The listing builds one solid part. Answer for the finished solid, in the listing's coordinates (mm). Face numbers are marked on the shaded views. A direction names the side the tool comes from. Give positions to 0.01 mm unless a question says otherwise; leave off trailing zeros. Order: outer loops, then holes, each group sorted by start corner. A loop starts at its lowest first (then second) coordinate and runs counter-clockwise, first axis right, second up. Notation, with made-up numbers: (45, -28.75) - (92, -28.75) arc R13 ccw to (92, -23.75) - close; hole circle Ø8 at (63, 46). An arc over 180 degrees is marked (long way). Use a Markdown table: item, result. Add a question column.
1) Flat-ended cylindrical pins translate along their axes: pin 1 (1 mm diameter, centred on y = 13, z = 19.5, fed in from +X); pin 2 (2.5 mm diameter, centred on x = 11.67, y = 11.67, fed in from -Z); pin 3 (4 mm diameter, centred on x = -11.5, z = 7, fed in from +Y). Find the tip coordinate at first contact, or state that the pin passes through.
2) Find section A-A, the plane z = 42. Determine the outline of the cut face in (x, y), plus the area to 3 significant figures.
3) The mould has two halves that part along Z. Classify the marked faces 4, 5 and 6: released by +Z, released by -Z, zero draft, split by the parting line, or undercut.
4) For the marked faces 1, 2 and 3, determine the directions among +Z, -Z, +X, -X, +Y, -Y from which every point of the face is accessible in a straight line to the end or side of a thin tool.
5) Find section B-B, the plane y = 0. Determine the outline of the cut face in (x, z).
6) Straight lines are drawn through the part: line 1 (Z direction, x = -1, y = -3); line 2 (X direction, y = -14, z = 58.1); line 3 (X direction, y = 10, z = 43.5). For each, find the intervals that lie inside material, in ascending order.
from build123d import *

# Parameters (mm, degrees)
SKETCH1_R           = 19
SKETCH1_R_2         = 1
BOSS_EXTRUDE1_DEPTH = 1.6
SKETCH2_R           = 19
SKETCH2_R_2         = 0.75
BOSS_EXTRUDE2_DEPTH = 6
SKETCH8_R           = 12.75
CUT_EXTRUDE4_DEPTH  = 1
SKETCH3_R           = 4.9
CUT_EXTRUDE1_DEPTH  = 6
BOSS_EXTRUDE3_DEPTH = 2
FILLET1_R           = 5
FILLET2_R           = 2
SKETCH5_W           = 5
SKETCH5_H           = 2.8
BOSS_EXTRUDE4_DEPTH = 6
SKETCH6_R           = 1.05
CUT_EXTRUDE2_DEPTH  = 72.802576555
SKETCH7_R           = 2
CUT_EXTRUDE3_DEPTH  = 1.5
FILLET3_R           = 2.5
FILLET4_R           = 2.5
FILLET5_R           = 1.5
FILLET6_R           = 2
BOSS_EXTRUDE5_START = 3
BOSS_EXTRUDE5_DEPTH = 3
FILLET8_R           = 1
SKETCH10_W          = 35
SKETCH10_H          = 19
CUT_EXTRUDE5_DEPTH  = 67.890657074
FILLET9_R           = 2
FILLET10_R          = 0.4


with BuildPart() as part:
    # Sketch1 → Boss-Extrude1 (new body)
    with BuildSketch(Plane.XY):
        Circle(SKETCH1_R)
        with Locations((-11.66726189, 11.66726189)):
            Circle(SKETCH1_R_2, mode=Mode.SUBTRACT)
        with Locations((11.66726189, 11.66726189)):
            Circle(SKETCH1_R_2, mode=Mode.SUBTRACT)
        with Locations((11.66726189, -11.66726189)):
            Circle(SKETCH1_R_2, mode=Mode.SUBTRACT)
        with Locations((-11.66726189, -11.66726189)):
            Circle(SKETCH1_R_2, mode=Mode.SUBTRACT)
    extrude(amount=BOSS_EXTRUDE1_DEPTH)

    # Sketch2 → Boss-Extrude2 (add)
    with BuildSketch(Plane.XY.offset(1.6)):
        Circle(SKETCH2_R)
        with Locations((-11.66726189, -11.66726189)):
            Circle(SKETCH2_R_2, mode=Mode.SUBTRACT)
        with Locations((-11.66726189, 11.66726189)):
            Circle(SKETCH2_R_2, mode=Mode.SUBTRACT)
        with Locations((11.66726189, 11.66726189)):
            Circle(SKETCH2_R_2, mode=Mode.SUBTRACT)
        with Locations((11.66726189, -11.66726189)):
            Circle(SKETCH2_R_2, mode=Mode.SUBTRACT)
    extrude(amount=BOSS_EXTRUDE2_DEPTH)

    # Sketch8 → Cut-Extrude4 (cut)
    with BuildSketch(Plane(origin=(0, 0, 0), x_dir=(-1, 0, 0), z_dir=(0, 0, -1))):
        Circle(SKETCH8_R)
    extrude(amount=-CUT_EXTRUDE4_DEPTH, mode=Mode.SUBTRACT)

    # Sketch3 → Cut-Extrude1 (cut)
    with BuildSketch(Plane.XY.offset(7.6)):
        Circle(SKETCH3_R)
    extrude(amount=-CUT_EXTRUDE1_DEPTH, mode=Mode.SUBTRACT)

    # Sketch4 → Boss-Extrude3 (add, symmetric)
    with BuildSketch(Plane(origin=(0, 0, 0), x_dir=(0, 0, -1), z_dir=(1, 0, 0))):
        Polygon((-7.6, 14.5), (-60.6, 14.5), (-60.6, -14.5), (-7.6, -14.5), (-7.6, -7), (-15.6, -7), (-15.6, 7), (-7.6, 7), align=None)
    extrude(amount=BOSS_EXTRUDE3_DEPTH, both=True)

    # Fillet1
    fillet1_edges = [part.edges().sort_by_distance(p)[0] for p in [
        (-2, 10.75, 7.6),
        (-2, -10.75, 7.6),
        (2, 10.75, 7.6),
        (2, -10.75, 7.6),
    ]]
    fillet(fillet1_edges, radius=FILLET1_R)

    # Fillet2
    fillet2_edges = [part.edges().sort_by_distance(p)[0] for p in [
        (0, -7, 15.6),
        (0, 7, 15.6),
    ]]
    fillet(fillet2_edges, radius=FILLET2_R)

    # Sketch5 → Boss-Extrude4 (add)
    with BuildSketch(Plane(origin=(-2, 14.5, 12.6), x_dir=(0, 0, -1), z_dir=(1, 0, 0))):
        with Locations((-45.5, -1.4)):
            Rectangle(SKETCH5_W, SKETCH5_H)
        with Locations((-6.5, -1.4)):
            Rectangle(SKETCH5_W, SKETCH5_H)
        with Locations((-6.5, -27.6)):
            Rectangle(SKETCH5_W, SKETCH5_H)
        with Locations((-45.5, -27.6)):
            Rectangle(SKETCH5_W, SKETCH5_H)
    extrude(amount=-BOSS_EXTRUDE4_DEPTH)

    # Sketch6 → Cut-Extrude2 (cut, through all)
    with BuildSketch(Plane(origin=(0, 14.5, 0), x_dir=(1, 0, 0), z_dir=(0, 1, 0))):
        with Locations(Location((-5.5, -58.1, 0), (0, 0, 270))):
            Circle(SKETCH6_R)
        with Locations(Location((-5.5, -19.1, 0), (0, 0, 270))):
            Circle(SKETCH6_R)
    extrude(amount=-CUT_EXTRUDE2_DEPTH, mode=Mode.SUBTRACT)

    # Sketch7 → Cut-Extrude3 (cut)
    with BuildSketch(Plane(origin=(0, 14.5, 0), x_dir=(1, 0, 0), z_dir=(0, 1, 0))):
        with Locations(Location((-5.5, -19.1, 0), (0, 0, 270))):
            Circle(SKETCH7_R)
        with Locations(Location((-5.5, -58.1, 0), (0, 0, 270))):
            Circle(SKETCH7_R)
    cut_extrude3 = extrude(amount=-CUT_EXTRUDE3_DEPTH, mode=Mode.SUBTRACT)

    # Mirror1: Cut-Extrude3 across plane
    add(cut_extrude3.mirror(Plane.ZX), mode=Mode.SUBTRACT)

    # Fillet3
    fillet3_edges = [part.edges().sort_by_distance(p)[0] for p in [
        (-8, -13.1, 60.6),
        (-8, -13.1, 55.6),
        (-8, 13.1, 60.6),
        (-8, 13.1, 55.6),
        (-8, -13.1, 21.6),
        (-8, -13.1, 16.6),
        (-8, 13.1, 21.6),
        (-8, 13.1, 16.6),
    ]]
    fillet(fillet3_edges, radius=FILLET3_R - 0.0001)  # a hair under: the kernel refuses the full size

    # Fillet4
    fillet4_edges = [part.edges().sort_by_distance(p)[0] for p in [
        (2, 0, 60.6),
    ]]
    fillet(fillet4_edges, radius=FILLET4_R)

    # Fillet5
    fillet5_edges = [part.edges().sort_by_distance(p)[0] for p in [
        (0, 14.5, 7.6),
        (0, -14.5, 7.6),
    ]]
    fillet(fillet5_edges, radius=FILLET5_R)

    # Fillet6
    fillet6_edges = [part.edges().sort_by_distance(p)[0] for p in [
        (0, 7, 7.6),
        (0, -7, 7.6),
    ]]
    fillet(fillet6_edges, radius=FILLET6_R)

    # Sketch9 → Boss-Extrude5 (add)
    with BuildSketch(Plane(origin=(0, 0, 0), x_dir=(-1, 0, 0), z_dir=(0, 0, -1)).offset(BOSS_EXTRUDE5_START)):
        with BuildLine():
            Line((-1, 18.973665961), (-1, 14.973665961))
            Line((-1, 14.973665961), (1, 14.973665961))
            Line((1, 14.973665961), (1, 18.973665961))
            ThreePointArc((1, 18.973665961), (0, 19), (-1, 18.973665961))
        make_face()
    extrude(amount=-BOSS_EXTRUDE5_DEPTH)

    # Fillet8
    fillet8_edges = [part.edges().sort_by_distance(p)[0] for p in [
        (-19, 0, 7.6),
    ]]
    fillet(fillet8_edges, radius=FILLET8_R)

    # Sketch10 → Cut-Extrude5 (cut, through all)
    with BuildSketch(Plane.ZY.offset(2)):
        with Locations((38.1, 0)):
            Rectangle(SKETCH10_W, SKETCH10_H)
    extrude(amount=-CUT_EXTRUDE5_DEPTH, mode=Mode.SUBTRACT)

    # Fillet9
    fillet9_edges = [part.edges().sort_by_distance(p)[0] for p in [
        (0, 9.5, 20.6),
        (0, 9.5, 55.6),
        (0, -9.5, 55.6),
        (0, -9.5, 20.6),
    ]]
    fillet(fillet9_edges, radius=FILLET9_R)

    # Fillet10
    fillet10_edges = [part.edges().sort_by_distance(p)[0] for p in [
        (1, 16.973665961, -3),
        (0, 14.973665961, -3),
        (-1, 16.973665961, -3),
        (0, 19, -3),
    ]]
    fillet(fillet10_edges, radius=FILLET10_R)


solid = part.part
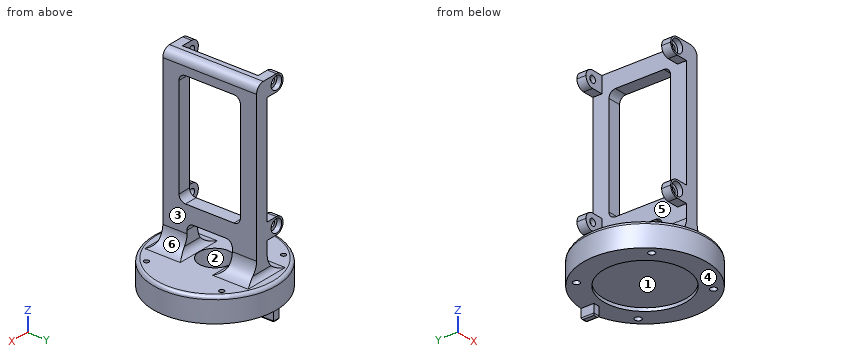
The answers:
| question | item | result |
|---|---|---|
| 1 | pin 1 | x = 2 |
| 1 | pin 2 | z = 0 |
| 1 | pin 3 | y = 16.44 |
| 2 | outline | (-2, -14.5) - (2, -14.5) - (2, -9.5) - (-2, -9.5) - close; (-2, 9.5) - (2, 9.5) - (2, 14.5) - (-2, 14.5) - close |
| 2 | area | 40.0 mm2 |
| 3 | face 4 | released by -Z |
| 3 | face 5 | undercut |
| 3 | face 6 | released by +Z |
| 4 | face 1 | -Z |
| 4 | face 2 | none |
| 4 | face 3 | +Z, +X, +Y, -Y |
| 5 | outline | (-19, 0) - (-12.75, 0) - (-12.75, 1) - (12.75, 1) - (12.75, 0) - (19, 0) - (19, 6.6) arc R1 ccw to (18, 7.6) - (4.9, 7.6) - (4.9, 1.6) - (-4.9, 1.6) - (-4.9, 7.6) - (-18, 7.6) arc R1 ccw to (-19, 6.6) - close; (-2, 15.6) - (2, 15.6) - (2, 20.6) - (-2, 20.6) - close; (-2, 55.6) - (2, 55.6) - (2, 58.1) arc R2.5 ccw to (-0.5, 60.6) - (-2, 60.6) - close |
| 6 | line 1 | 1 to 1.6, 15.6 to 20.6, 55.6 to 60.6 |
| 6 | line 2 | -8 to -7.5, -3.5 to 2 |
| 6 | line 3 | -2 to 2 |
